from build123d import *

# Parameters (mm, degrees)
F0_W     = 254
F0_H     = 355.6
F1_DEPTH = 254
F2_R     = 5.08
F3_R     = 61.292809
F4_DEPTH = 254.001
F5_SIZE  = 5.08


with BuildPart() as f1:
    # F0 (on Top) → F1 (new body)
    with BuildSketch(Plane.XY):
        with Locations((127, 177.8)):
            Rectangle(F0_W, F0_H)
    extrude(amount=F1_DEPTH)

    # F2
    f2_edges = [f1.edges().sort_by_distance(p)[0] for p in [
        (254, 0, 127),
        (254, 355.6, 127),
        (0, 0, 127),
        (0, 177.8, 0),
        (127, 355.6, 0),
        (127, 0, 0),
        (254, 177.8, 0),
        (0, 355.6, 127),
        (0, 177.8, 254),
        (127, 355.6, 254),
        (254, 177.8, 254),
        (127, 0, 254),
    ]]
    fillet(f2_edges, radius=F2_R)

    # F3 (on face) → F4 (cut, through all)
    with BuildSketch(Plane.XY.offset(254)):
        with Locations((123.2237, 104.999602)):
            Circle(F3_R)
    extrude(amount=-F4_DEPTH, mode=Mode.SUBTRACT)

    # F5
    f5_edges = [f1.edges().sort_by_distance(p)[0] for p in [
        (61.930891, 104.999602, 254),
        (61.930891, 104.999602, 0),
    ]]
    chamfer(f5_edges, length=F5_SIZE)


solid = f1.part
Geometry check sheet. Reference: the model listing, model coordinates, mm. Coordinates: 2 decimals unless noted, no trailing zeros. Order: outer loops, then holes, each group sorted by start corner. A loop starts at its lowest first (then second) coordinate and runs counter-clockwise, first axis right, second up. Notation, with made-up numbers: (71.25, 76.5) -> (83.25, 76.5) arc R20 cw to (83.25, 80.5) -> close; hole circle Ø5 at (48, -36). An arc over 180 degrees is marked (long way). Use a Markdown table: item, result. Add a question column.
1. Cross-section at A-A (z = 32.5). Enter the section's corners in (x, y).
2. Mould release check, pull along X, two halves, no side actions. Record for faces 1 (the face through (109.88, 44.92, 249.17)), 2 (the face through (125, 0, 125)), 3 (the face through (254, 175, 125)): pulls with the +X half, pulls with the -X half, needs draft (parallel to the pull), parting line crosses it, or undercut.
3. Material ranges on L1, parallel to X at y = 120.5, z = 227; L2, parallel to Y at x = 115, z = 202.5; L3, parallel to Y at x = 136, z = 86, recorded low to high.
Filled sheet:
| question | item | result |
|---|---|---|
| 1 | outline | (0, 5.08) arc R5.08 ccw to (5.08, 0) -> (248.92, 0) arc R5.08 ccw to (254, 5.08) -> (254, 350.52) arc R5.08 ccw to (248.92, 355.6) -> (5.08, 355.6) arc R5.08 ccw to (0, 350.52) -> close; hole circle Ø122.59 at (123.22, 105) |
| 2 | face 1 | undercut |
| 2 | face 2 | needs draft |
| 2 | face 3 | pulls with the +X half |
| 3 | L1 | 0 to 63.92, 182.52 to 254 |
| 3 | L2 | 0 to 44.26, 165.74 to 355.6 |
| 3 | L3 | 0 to 45.05, 164.95 to 355.6 |
